Autodesk Inventor part; units mm, degrees
ref_plane "YZ Plane" through (0, 0, 0) normal (1, 0, 0) x (0, 1, 0)
ref_plane "XZ Plane" through (0, 0, 0) normal (0, 1, 0) x (-1, 0, 0)
ref_plane "XY Plane" through (0, 0, 0) normal (0, 0, 1) x (1, 0, 0)
sketch "Náčrt1" plane through (0, 0, 0) normal (0, 1, 0) x (1, 0, 0)
  line L0 (-250, 0) -> (250, 0)
  line L1 (250, 0) -> (100, -600)
  line L2 (100, -600) -> (100, -650)
  line L3 (100, -650) -> (-100, -650)
  line L4 (-100, -650) -> (-100, -600)
  line L5 (-100, -600) -> (-250, 0)
  point P0 (0, 0)
  point P1 (0, 0)
  point P2 (0, -650)
  dimension "d0" = 500
  dimension "d1" = 50
  dimension "d2" = 600
  dimension "d3" = 200
extrude "Vysunutí1" add sketch "Náčrt1" along normal blind 2800
sketch "Náčrt2" plane through (-100, 0, 650) normal (0, 0, 1) x (1, 0, 0)
  line L0 (200, 0) -> (0, 0) construction
  line L1 (200, 0) -> (200, 2800) construction
  circle A0 centre (100, 100) radius 25
  circle A1 centre (100, 2700) radius 35.9949 construction
  line L2 (100, 100) -> (100, 2700) construction
  point P0 (100, 0)
  point P1 (100, 1400)
  point P2 (200, 1400)
  point P3 (100, 0)
  dimension "d6" = 2600
  dimension "d7" = 50
extrude "Vysunutí2" cut sketch "Náčrt2" against normal blind 100
pattern_linear "Obdélníkové pole1" count 14 spacing 200 along (0, 1, 0) of "Vysunutí2"
properties part number "22002102_Suppot Beam"
Design review of the part built by this model. Coordinates are the model's own, in mm. A direction names the side the tool comes from. Round coordinates to 2 decimals unless told otherwise and drop trailing zeros. Write each loop counter-clockwise with the first axis right and the second up, starting at its lowest first coordinate (ties: lowest second). Pieces come first, ordered by that corner, then holes. Notation, with made-up numbers: (54.25, 76) -> (107.25, 76) arc R18 ccw to (107.25, 95) -> close; hole circle Ø7 at (-16.75, 46.5). An arc over 180 degrees is marked (long way). One line per item, written item: value. Start each with the question number.
Q1. Add section B-B (x = -195.5). Give the boundary of the cut face in (y, z).
Q2. Add section C-C (z = 511). Give the boundary of the cut face in (x, y).
Q3. Insertion check: P1, Ø25, axis at y = 1499.5, z = 634.5, coming from the +X side; P2, Ø4, axis at y = 2276, z = 559, coming from the -X side; P3, Ø1.5, axis at y = 323.5, z = 475, coming from the -X side; P4, Ø2, axis at x = 9, y = 1602, coming from the -Z side. Each pin has a flat end and moves straight along its axis. Give the tip position at first contact, or say it passes through.
Q4. Add section A-A (y = 1377.5). Give the boundary of the cut face in (x, z), then the cut area to 3 significant figures.
Q5. To check wall thickness, follow probe 1 along X at (y, z) = (2300, 618); probe 2 along X at (y, z) = (2700, 576); probe 3 along X at (y, z) = (2332.5, 155). State the ranges of each line that lie inside material, in increasing order.
Q6. Tool access review of faces 4 (the face through (1, 1380, 650)), 5 (the face through (0, 900, 550)), 6 (the face through (100, 1380, 625)), 7 (the face through (-100, 1380, 625)): name each direction out of +Z, -Z, +X, -X, +Y, -Y from which nothing blocks a thin tool from reaching the whole face with its end or side.
Q7. The part is to be moulded in two halves that separate along Y. For faces 1 (the face through (-3.255, 524.787, 600.7)), 2 (the face through (-174, 1380, 304)), 3 (the face through (-4, 2800, 248)), say which applies: pulls with the +Y half, pulls with the -Y half, needs draft (parallel to the pull), parting line crosses it, or undercut.
Response:
1. outline: (0, 0) -> (2800, 0) -> (2800, 218) -> (0, 218) -> close
2. outline: (-122.25, 0) -> (122.25, 0) -> (122.25, 2800) -> (-122.25, 2800) -> close
3. P1: stops at x = 100
3. P2: stops at x = -110.75
3. P3: stops at x = -131.44
3. P4: stops at z = 0
4. outline: (-250, 0) -> (250, 0) -> (100, 600) -> (100, 650) -> (-100, 650) -> (-100, 600) -> close
4. area: 220,000 mm^2
5. probe 1: x = -100 to -25, 25 to 100
5. probe 2: x = -106 to -25, 25 to 106
5. probe 3: x = -211.25 to 211.25
6. face 4: +Z, +X, -X, +Y, -Y
6. face 5: +Z
6. face 6: +Z, +X, +Y, -Y
6. face 7: +Z, -X, +Y, -Y
7. face 1: undercut
7. face 2: needs draft
7. face 3: pulls with the +Y half
